Autodesk Fusion 360 part; units mm, degrees
sketch "Sketch1" plane through (0, 0, 0) normal (0, 1, 0) x (1, 0, 0)
  line L0 (-7.5, 0) -> (-6, 0)
  line L1 (-6, 0) -> (-6, -7.5)
  line L2 (-4, -9.5) -> (4, -9.5)
  line L3 (6, -7.5) -> (6, 0)
  line L4 (6, 0) -> (7.5, 0)
  line L5 (7.5, 0) -> (7.5, -10)
  line L6 (6.5, -11) -> (-6.5, -11)
  line L7 (-7.5, -10) -> (-7.5, 0)
  line L8 (0, 0) -> (0, -11)
  arc A0 (-6, -7.5) -> (-4, -9.5) centre (-4, -7.5) ccw
  arc A1 (4, -9.5) -> (6, -7.5) centre (4, -7.5) ccw
  arc A2 (-7.5, -10) -> (-6.5, -11) centre (-6.5, -10) ccw
  arc A3 (6.5, -11) -> (7.5, -10) centre (6.5, -10) ccw
  point P0 (-6, -9.5)
  point P1 (7.5, -11)
  point P2 (-7.5, -11)
  dimension "d2" = 15
  dimension "d3" = 1.5
  dimension "d6" = 2
  dimension "d7" = 2
  dimension "d8" = 1.5
  dimension "d9" = 1
  dimension "d10" = 1
  dimension "d11" = 11
extrude "Extrude1" add sketch "Sketch1" along normal mid plane 11.5
sketch "Sketch2" plane through (0, 0, 0) normal (0, 0, 1) x (1, 0, 0)
  line L0 (-7.5, -5.75) -> (-7.5, 5.75)
  line L1 (-6, -5.75) -> (-6, 5.75)
  line L2 (6, -5.75) -> (6, 5.75)
  line L3 (7.5, -5.75) -> (7.5, 5.75)
  line L4 (-7.5, 2.75) -> (7.5, 2.75) construction
  line L5 (7.5, -5.75) -> (9.4843, -5.75)
  line L6 (7.5, 2.75) -> (9.4843, 2.75)
  line L7 (-7.5, 2.75) -> (-9.4843, 2.75)
  line L8 (-7.5, -5.75) -> (-9.4843, -5.75)
  arc A0 (-10.8072, 2.25) -> (-10.8072, -5.25) centre (-7.5, -1.5) ccw
  arc A1 (10.8072, -5.25) -> (10.8072, 2.25) centre (7.5, -1.5) ccw
  line L9 (12.5, -5.75) -> (12.5, 2.75) construction
  line L10 (-12.5, -5.75) -> (-12.5, 2.75) construction
  arc A2 (-10.8072, -5.25) -> (-9.4843, -5.75) centre (-9.4843, -3.75) ccw
  arc A3 (-9.4843, 2.75) -> (-10.8072, 2.25) centre (-9.4843, 0.75) ccw
  arc A4 (10.8072, 2.25) -> (9.4843, 2.75) centre (9.4843, 0.75) ccw
  arc A5 (9.4843, -5.75) -> (10.8072, -5.25) centre (9.4843, -3.75) ccw
  dimension "d15" = 3
  dimension "d16" = 5
  dimension "d17" = 25
  dimension "d18" = 2
extrude "Extrude2" add sketch "Sketch2" along normal blind 3
fillet "Fillet1" radius 1 2 edges at (7.5, -1.5, 3) (-7.5, -1.5, 3)
sketch "Sketch3" plane through (0, 0, 0) normal (0, 0, -1) x (1, 0, 0)
  line L0 (6, 5.75) -> (6, -5.75)
  line L1 (6, -5.75) -> (7.5, -5.75)
  line L2 (7.5, -5.75) -> (7.5, -2.75)
  line L3 (7.5, -2.75) -> (9.4843, -2.75)
  arc A0 (9.4843, -2.75) -> (10.8072, -2.25) centre (9.4843, -0.75) ccw
  arc A1 (10.8072, -2.25) -> (10.8072, 5.25) centre (7.5, 1.5) ccw
  arc A2 (10.8072, 5.25) -> (9.4843, 5.75) centre (9.4843, 3.75) ccw
  line L4 (9.4843, 5.75) -> (6, 5.75)
  line L5 (6, 5.75) -> (6, -5.75)
  line L6 (7.5, -2.75) -> (7.5, -5.75)
  line L7 (9, 2.5) -> (7.5, 2.5)
  line L8 (7.5, 0.5) -> (9, 0.5)
  arc A3 (9, 0.5) -> (9, 2.5) centre (9, 1.5) ccw
  line L9 (7.5, -2.75) -> (7.5, 5.75) construction
  line L10 (7.5, 2.5) -> (7.5, 3)
  line L11 (7.5, 3) -> (6, 3)
  line L12 (7.5, 0.5) -> (7.5, 0)
  line L13 (7.5, 0) -> (6, 0)
  arc A4 (10.8072, -2.25) -> (10.8072, 5.25) centre (7.5, 1.5) ccw
  dimension "d24" = 2
  dimension "d25" = 0.5
  dimension "d26" = 1.5
extrude "Extrude3" cut sketch "Sketch3" against normal blind 1 contours L0 L5 L7 L8 A3 L10 L11 L12 L13
mirror "Mirror1" about plane through (0, 0, 0) normal (1, 0, 0) of "Extrude3"
sketch "Sketch4" plane through (0, 0, 1) normal (0, 0, -1) x (1, 0, 0)
  line L0 (-9, 0.5) -> (-7.5, 0.5)
  line L1 (-7.5, 0.5) -> (-7.5, 0)
  line L2 (-7.5, 0) -> (-6, 0)
  line L3 (-6, 0) -> (-6, 3)
  line L4 (-6, 3) -> (-7.5, 3)
  line L5 (-7.5, 3) -> (-7.5, 2.5)
  line L6 (-7.5, 2.5) -> (-9, 2.5)
  arc A0 (-9, 2.5) -> (-9, 0.5) centre (-9, 1.5) ccw
  line L7 (-6, 3) -> (-6, 0)
  line L8 (-6, 3) -> (-7.5, 3)
  line L9 (-7.5, 3) -> (-7.5, 2.5)
  line L10 (-7.5, 2.5) -> (-9, 2.5)
  arc A1 (-9, 2.5) -> (-9, 0.5) centre (-9, 1.5) ccw
  line L11 (-7.5, 0.5) -> (-7.5, 0)
  line L12 (-7.5, 3) -> (-6, 3)
  line L13 (-6, 3) -> (-6, 5.75)
  line L14 (-6, 5.75) -> (-9.4843, 5.75)
  arc A2 (-9.4843, 5.75) -> (-10.8072, 5.25) centre (-9.4843, 3.75) ccw
  arc A3 (-10.8072, 5.25) -> (-10.8072, -2.25) centre (-7.5, 1.5) ccw
  arc A4 (-10.8072, -2.25) -> (-9.4843, -2.75) centre (-9.4843, -0.75) ccw
  line L15 (-9.4843, -2.75) -> (-7.5, -2.75)
  line L16 (-7.5, -2.75) -> (-7.5, -5.75)
  line L17 (-7.5, -5.75) -> (-6, -5.75)
  line L18 (-6, -5.75) -> (-6, 0)
  line L19 (-6, 0) -> (-7.5, 0)
  line L20 (-7.5, 0) -> (-7.5, 0.5)
  line L21 (-7.5, 0.5) -> (-9, 0.5)
  arc A5 (-9, 2.5) -> (-9, 0.5) centre (-9, 1.5) ccw
  line L22 (-9, 2.5) -> (-7.5, 2.5)
  line L23 (-7.5, 2.5) -> (-7.5, 3)
  line L24 (-6, 0) -> (-7.5, 0)
  line L25 (-7.5, 3) -> (-6, 3)
  line L26 (-6, 3) -> (-6, 0)
  line L27 (-6, 0) -> (-7.5, 0)
  line L28 (-7.5, 0) -> (-7.5, 3)
extrude "Extrude4" cut sketch "Sketch4" against normal blind 2 contours L1 L2 L3 L4 L5 L7 L8 L9 L11 L12 L19 L20 L23 L24 L25 L26 L27 L28
mirror "Mirror2" about plane through (0, 0, 0) normal (1, 0, 0) of "Extrude4"
sketch "Sketch5" plane through (0, 0, 3) normal (0, 0, 1) x (-1, 0, 0)
  line L0 (-8.5, -2.75) -> (-8.5, 5.75)
  line L1 (-8.5, 5.75) -> (-9.4843, 5.75)
  arc A0 (-9.4843, 5.75) -> (-10.8072, 5.25) centre (-9.4843, 3.75) ccw
  arc A1 (-10.8072, 5.25) -> (-10.8072, -2.25) centre (-7.5, 1.5) ccw
  arc A2 (-10.8072, -2.25) -> (-9.4843, -2.75) centre (-9.4843, -0.75) ccw
  line L2 (-9.4843, -2.75) -> (-8.5, -2.75)
  line L3 (-9, -0.5) -> (-7.2679, 0.5)
  line L4 (-7.2679, 0.5) -> (-7.2679, 2.5)
  line L5 (-7.2679, 2.5) -> (-9, 3.5)
  line L6 (-9, 3.5) -> (-10.7321, 2.5)
  line L7 (-10.7321, 2.5) -> (-10.7321, 0.5)
  line L8 (-10.7321, 0.5) -> (-9, -0.5)
  arc A3 (-10.8072, 5.25) -> (-10.8072, -2.25) centre (-7.5, 1.5) ccw
  arc A4 (-9, 2.5) -> (-9, 0.5) centre (-9, 1.5) ccw
  point P0 (-9, 1.5)
  dimension "d35" = 2
extrude "Extrude5" cut sketch "Sketch5" along normal blind 1 and the other way blind 2 contours L0 L3 L5 L6 L7 L8 | L0 L3 L4 L5
mirror "Mirror3" about plane through (0, 0, 0) normal (1, 0, 0) of "Extrude5"
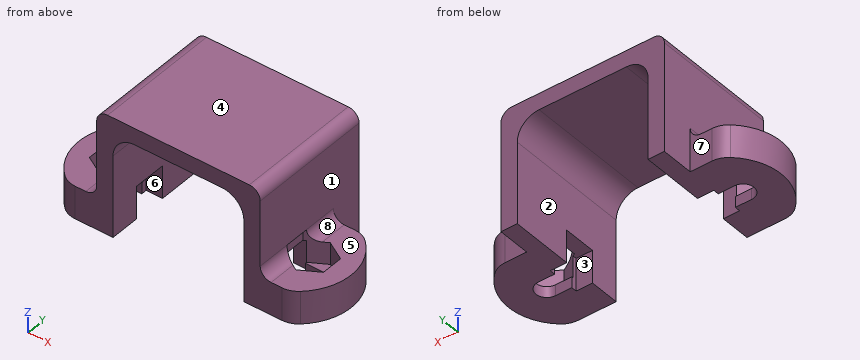
The model under review builds one solid part; all positions refer to its coordinate system, in mm. Face numbers are marked on the shaded views. A direction names the side the tool comes from. Round coordinates to 2 decimals unless told otherwise and drop trailing zeros. Order: outer loops, then holes, each group sorted by start corner. A loop starts at its lowest first (then second) coordinate and runs counter-clockwise, first axis right, second up. Notation, with made-up numbers: (21, 50.5) - (43, 50.5) arc R15 ccw to (43, 63.5) - close; hole circle Ø3 at (68, 42.25). An arc over 180 degrees is marked (long way). Use one line per item in the form item = value.
Q1. To check wall thickness, follow line 1 (X direction, y = 3.25, z = 4.75); line 2 (X direction, y = -2, z = 3.25); line 3 (Z direction, x = -3.5, y = 1.75). State the ranges of each line that lie inside material, in increasing order.
Response values:
line_1 = -7.5 to -6, 6 to 7.5
line_2 = -7.27 to -6, 6 to 7.27
line_3 = 9.5 to 11
Q2. Add section D-D on y = 3.25. Give the boundary of the cut face in (x, z).
Response values:
outline = (-7.5, 0) - (-6, 0) - (-6, 7.5) arc R2 cw to (-4, 9.5) - (4, 9.5) arc R2 cw to (6, 7.5) - (6, 0) - (7.5, 0) - (7.5, 10) arc R1 ccw to (6.5, 11) - (-6.5, 11) arc R1 ccw to (-7.5, 10) - close
Q3. Mouldability with a two-part tool opening along Y and no side actions: class the marked faces 6, 7 and 8 as pulls with the +Y half, pulls with the -Y half, needs draft (parallel to the pull), parting line crosses it, or undercut.
Response values:
face_6 = undercut
face_7 = pulls with the +Y half
face_8 = needs draft
Q4. Add section B-B on y = -1.5. Give the boundary of the cut face in (x, z), then the cut area to 3 significant figures.
Response values:
outline = (-12.5, 0) - (-10, 0) - (-10, 1) - (-10.73, 1) - (-10.73, 3) - (-12.5, 3) - close; (-7.5, 4) - (-7.27, 4) - (-7.27, 3) - (-6, 3) - (-6, 7.5) arc R2 cw to (-4, 9.5) - (4, 9.5) arc R2 cw to (6, 7.5) - (6, 3) - (7.27, 3) - (7.27, 4) - (7.5, 4) - (7.5, 10) arc R1 ccw to (6.5, 11) - (-6.5, 11) arc R1 ccw to (-7.5, 10) - close; (10, 0) - (12.5, 0) - (12.5, 3) - (10.73, 3) - (10.73, 1) - (10, 1) - close
area = 54.9 mm^2
Q5. Clearance check with flat-ended pins moving along their axes: P1, Ø3, axis at y = 4, z = 8.5, coming from the -X side; P2, Ø1.2, axis at x = -10.5, y = -2, coming from the +Z side; P3, Ø1, axis at x = 8.5, y = 4.5, coming from the -Z side; P4, Ø1, axis at y = -3, z = 6.5, coming from the +X side. State where each tip first meets the part, or that it passes through.
Response values:
P1 = -7.5
P2 = 3
P3 = through
P4 = 7.5
Q6. Tool access review of the marked faces 1, 2, 3, 4 and 5: name each direction out of +Z, -Z, +X, -X, +Y, -Y from which nothing blocks a thin tool from reaching the whole face with its end or side.
Response values:
face_1 = +Z, +X, +Y
face_2 = -Z, +Y, -Y
face_3 = -Z
face_4 = +Z, +X, -X, +Y, -Y
face_5 = +Z, +X, +Y, -Y
Q7. Add section A-A on z = 4.75. Give the boundary of the cut face in (x, y), then the cut area to 3 significant figures.
Response values:
outline = (-7.5, -5.75) - (-6, -5.75) - (-6, 5.75) - (-7.5, 5.75) - close; (6, -5.75) - (7.5, -5.75) - (7.5, 5.75) - (6, 5.75) - close
area = 34.5 mm^2
Q8. Add section C-C on x = 8. Give the boundary of the cut face in (y, z), then the cut area to 3 significant figures.
Response values:
outline = (-5.75, 0) - (-2.5, 0) - (-2.5, 1) - (-2.92, 1) - (-2.92, 3.13) - (-5.75, 3.13) - close; (-0.5, 0) - (2.75, 0) - (2.75, 3.13) - (-0.08, 3.13) - (-0.08, 1) - (-0.5, 1) - close
area = 18.6 mm^2
